Read the model definition and answer for the solid it produces. Units are mm, in the model's axes. A direction names the side the tool comes from. Coordinates: 2 decimals unless noted, no trailing zeros. Order: outer loops, then holes, each group sorted by start corner. A loop starts at its lowest first (then second) coordinate and runs counter-clockwise, first axis right, second up.
```python
from build123d import *

# Parameters (mm, degrees)
SKETCH_W               = 45
SKETCH_H               = 20
PAD_DEPTH              = 3
SKETCH001_R            = 1
POCKET_DEPTH           = 5
POLARPATTERN_COUNT     = 2
SKETCH002_R            = 8
PAD001_DEPTH           = 13.3
POLARPATTERN001_COUNT  = 2
PAD002_DEPTH           = 3.5
SKETCH006_W            = 10.16
SKETCH006_H            = 2.54
PAD003_DEPTH           = 2
SKETCH007_W            = 0.707106
SKETCH007_H            = 0.707106
PAD004_DEPTH           = 2
LINEARPATTERN_COUNT    = 4
LINEARPATTERN_PITCH    = 2.54
SKETCH008_W            = 0.707106
SKETCH008_H            = 0.707107
PAD005_DEPTH           = 6.5
LINEARPATTERN001_COUNT = 4
LINEARPATTERN001_PITCH = 2.54
SKETCH009_R            = 1
POCKET001_DEPTH        = 5
POLARPATTERN002_COUNT  = 2
SKETCH010_R            = 6.5
POCKET002_DEPTH        = 0.5
POLARPATTERN003_COUNT  = 2


with BuildPart() as part:
    # Sketch → Pad (new body)
    with BuildSketch(Plane.XY):
        Rectangle(SKETCH_W, SKETCH_H)
    extrude(amount=PAD_DEPTH)

    # Sketch001 (on Face6 of Pad) → Pocket (cut)
    with BuildSketch(Plane.XY.offset(3)):
        with Locations((20, 7.5)):
            Circle(SKETCH001_R)
    pocket = extrude(amount=-POCKET_DEPTH, mode=Mode.SUBTRACT)

    # PolarPattern: Pocket ×2 about axis
    polarpattern_axis = Axis((0, 0, 3), (0, 0, 1))
    for i in range(1, POLARPATTERN_COUNT):
        add(pocket.rotate(polarpattern_axis, i * 360 / POLARPATTERN_COUNT), mode=Mode.SUBTRACT)

    # Sketch002 (on Face5 of PolarPattern) → Pad001 (join)
    with BuildSketch(Plane.XY.offset(3)):
        with Locations((13.5, 0)):
            Circle(SKETCH002_R)
    pad001 = extrude(amount=PAD001_DEPTH)

    # PolarPattern001: Pad001 ×2 about axis
    polarpattern001_axis = Axis((0, 0, 3), (0, 0, 1))
    for i in range(1, POLARPATTERN001_COUNT):
        add(pad001.rotate(polarpattern001_axis, i * 360 / POLARPATTERN001_COUNT))

    # Sketch003 (on Face5 of PolarPattern001) → Pad002 (join)
    with BuildSketch(Plane.XY.offset(3)):
        with BuildLine():
            ThreePointArc((-3.125, -5), (-5.375, -7.25), (-3.125, -9.5))
            Line((-3.125, -9.5), (3.125, -9.5))
            ThreePointArc((3.125, -9.5), (5.375, -7.25), (3.125, -5))
            Line((-3.125, -5), (3.125, -5))
        make_face()
    extrude(amount=PAD002_DEPTH)

    # Sketch006 (on Face4 of Pad002) → Pad003 (join)
    with BuildSketch(Plane(origin=(0, 0, 0), x_dir=(1, 0, 0), z_dir=(0, 0, -1))):
        with Locations((0, -8.73)):
            Rectangle(SKETCH006_W, SKETCH006_H)
    extrude(amount=PAD003_DEPTH)

    # Sketch007 (on Face13 of Pad003) → Pad004 (join)
    with BuildSketch(Plane(origin=(0, 0, -2), x_dir=(1, 0, 0), z_dir=(0, 0, -1))):
        with Locations((-3.81, -8.73)):
            Rectangle(SKETCH007_W, SKETCH007_H)
    pad004 = extrude(amount=PAD004_DEPTH)

    # LinearPattern: Pad004 ×4
    with Locations(*[(i * LINEARPATTERN_PITCH, 0, 0) for i in range(1, LINEARPATTERN_COUNT)]):
        add(pad004)

    # Sketch008 (on Face31 of LinearPattern) → Pad005 (join)
    with BuildSketch(Plane(origin=(0, 9.083553, 0), x_dir=(-1, 0, 0), z_dir=(0, 1, 0))):
        with Locations((-3.81, -3.646443)):
            Rectangle(SKETCH008_W, SKETCH008_H)
    pad005 = extrude(amount=PAD005_DEPTH)

    # LinearPattern001: Pad005 ×4
    with Locations(*[(-i * LINEARPATTERN001_PITCH, 0, 0) for i in range(1, LINEARPATTERN001_COUNT)]):
        add(pad005)

    # Sketch009 → Pocket001 (cut)
    with BuildSketch(Plane.XY.offset(3)):
        with Locations((20, -7.5)):
            Circle(SKETCH009_R)
    pocket001 = extrude(amount=-POCKET001_DEPTH, mode=Mode.SUBTRACT)

    # PolarPattern002: Pocket001 ×2 about axis
    polarpattern002_axis = Axis((0, 0, 3), (0, 0, 1))
    for i in range(1, POLARPATTERN002_COUNT):
        add(pocket001.rotate(polarpattern002_axis, i * 360 / POLARPATTERN002_COUNT), mode=Mode.SUBTRACT)

    # Sketch010 (on Face76 of PolarPattern002) → Pocket002 (cut)
    with BuildSketch(Plane.XY.offset(16.3)):
        with Locations((13.5, 0)):
            Circle(SKETCH010_R)
    pocket002 = extrude(amount=-POCKET002_DEPTH, mode=Mode.SUBTRACT)

    # PolarPattern003: Pocket002 ×2 about axis
    polarpattern003_axis = Axis((0, 0, 16.3), (0, 0, 1))
    for i in range(1, POLARPATTERN003_COUNT):
        add(pocket002.rotate(polarpattern003_axis, i * 360 / POLARPATTERN003_COUNT), mode=Mode.SUBTRACT)


solid = part.part
```
1) Which of the six approach directions +Z, -Z, +X, -X, +Y, -Y give full straight-line access (tool end or side, diameter ignored) to faces 4 (the flat face through (0.916, 11.2, -3.7)), 5 (the flat face through (0, -7, 6.5)), 6 (the cylindrical face through (7.151, -4.868, 9.557)), 7 (the flat face through (-4.164, 11.2, -3.7))?
A:
face 4: -Z, +Y, -Y
face 5: +Z, +Y, -Y
face 6: +Z
face 7: -Z, -X, +Y, -Y
2) A cutting plane is placed at D-D, the plane x = 13.5. Determine the outline of the cut face in (y, z).
A:
outline: (-10, 0) - (10, 0) - (10, 3) - (8, 3) - (8, 16.3) - (6.5, 16.3) - (6.5, 15.8) - (-6.5, 15.8) - (-6.5, 16.3) - (-8, 16.3) - (-8, 3) - (-10, 3) - close
3) Flat-ended cylindrical pins translate along their axes: pin 1 Ø8 at (y, z) = (10, 12.5) entering from -X; pin 2 Ø1.6 at (y, z) = (11.5, -3) entering from +X; pin 3 Ø1.5 at (x, z) = (-4.5, 5) entering from -Y. Find the tip coordinate at first contact, or state that the pin passes through.
A:
pin 1: stops at x = -18.79
pin 2: stops at x = 4.16
pin 3: stops at y = -9.41
4) Straight lines are drawn through the part: line 1 (Y direction, x = 20, z = 1); line 2 (Y direction, x = -13.5, z = 16.1); line 3 (Z direction, x = 4, y = -7.5). For each, find the intervals that lie inside material, in ascending order.
A:
line 1: y = -10 to -8.5, -6.5 to 6.5, 8.5 to 10
line 2: y = -8 to -6.5, 6.5 to 8
line 3: z = 0 to 6.5
5) A cutting plane is placed at A-A, the plane z = 1.5. Determine the outline of the cut face in (x, y).
A:
outline: (-22.5, -10) - (22.5, -10) - (22.5, 10) - (-22.5, 10) - close; hole circle Ø2 at (-20, -7.5); hole circle Ø2 at (-20, 7.5); hole circle Ø2 at (20, -7.5); hole circle Ø2 at (20, 7.5)
6) Determine the mould class of faces 1 (the flat face through (22.5, 0, 1)), 2 (the flat face through (0, 7.46, -1)), 3 (the flat face through (-3.456, 11.2, -3.7)) for opening direction X: pulls with the +X half, pulls with the -X half, needs draft (parallel to the pull), parting line crosses it, or undercut.
A:
face 1: pulls with the +X half
face 2: needs draft
face 3: undercut
7) A cutting plane is placed at B-B, the plane y = -7.5. Determine the outline of the cut face in (x, z).
A:
outline: (-22.5, 0) - (-21, 0) - (-21, 3) - (-22.5, 3) - close; (-19, 0) - (19, 0) - (19, 3) - (16.28, 3) - (16.28, 16.3) - (10.72, 16.3) - (10.72, 3) - (5.36, 3) - (5.36, 6.5) - (-5.36, 6.5) - (-5.36, 3) - (-10.72, 3) - (-10.72, 16.3) - (-16.28, 16.3) - (-16.28, 3) - (-19, 3) - close; (21, 0) - (22.5, 0) - (22.5, 3) - (21, 3) - close
8) A cutting plane is placed at C-C, the plane z = 11. Determine the outline of the cut face in (x, y).
A:
outline: circle Ø16 at (-13.5, 0); circle Ø16 at (13.5, 0)
